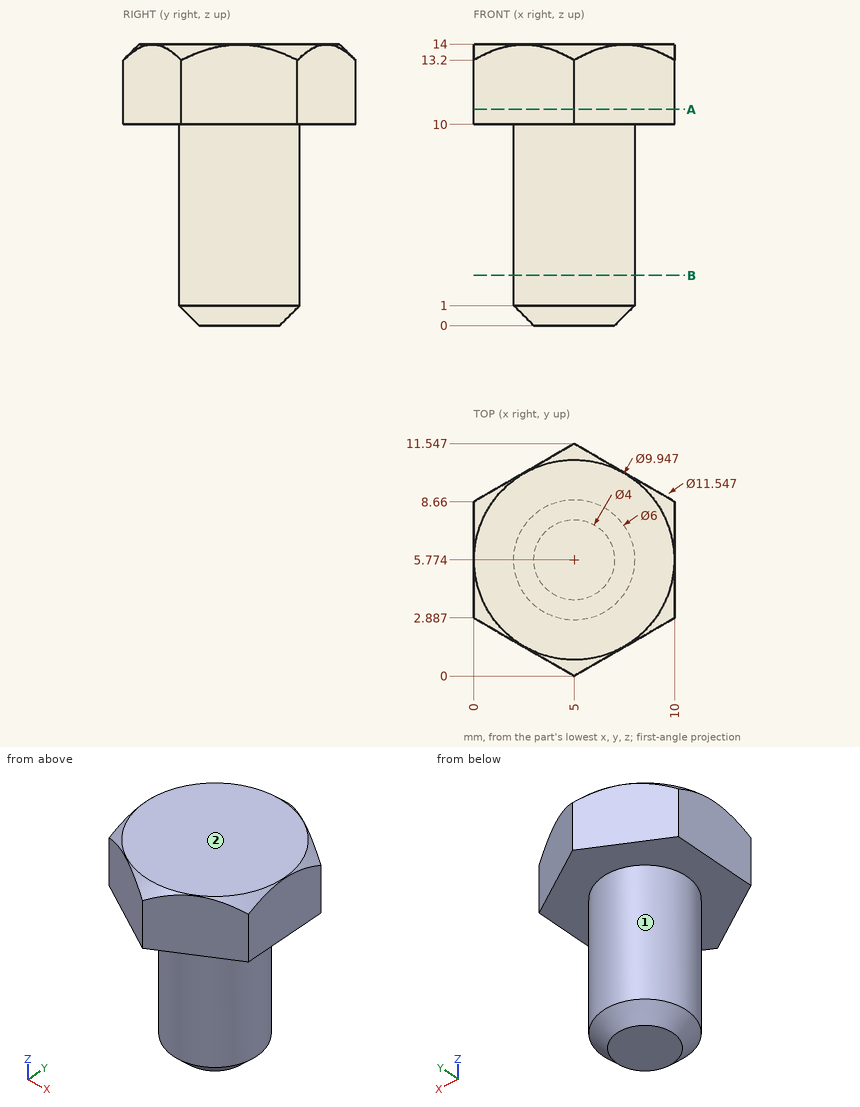
Source: three-view drawing plus pictorial views. Frame: mm from the lowest corner of the part. A direction names the side the tool comes from. Give positions to 0.01 mm unless a question says otherwise; leave off trailing zeros. Order: outer loops, then holes, each group sorted by start corner. A loop starts at its lowest first (then second) coordinate and runs counter-clockwise, first axis right, second up. Notation, with made-up numbers: (-24, 22) - (9, 22) arc R8 cw to (9, 32) - close; hole circle Ø5 at (8.5, 74.25). An arc over 180 degrees is marked (long way). Answer as a JSON object with one key per item and string values. Group by question number.
Q1. First-contact query: pin 1 Ø1 at (y, z) = (5.5, 6.5) entering from -X; pin 2 Ø2 at (x, y) = (2.5, 7.5) entering from -Z. Flat tips, straight axial feed; report the tip coordinate or a pass-through.
Q2. Cut plane A-A, the plane z = 10.75. Output: boundary loops of the cut face in (x, y).
Q3. Cut plane B-B, the plane z = 2.5. Output: boundary loops of the cut face in (x, y).
Q4. Line query: probe 1 along Z at (x, y) = (1, 5.75); probe 2 along Y at (x, z) = (5, 6.5); probe 3 along Y at (x, z) = (1.75, 12.75) (1 decimal). Output: solid intervals per line, ascending.
Q5. Set-up query: the marked faces 1 and 2. Return all of +Z, -Z, +X, -X, +Y, -Y with unobstructed straight access to the full face (end or side cutting, diameter ignored); none if empty.
Results:
{
 "1": {"pin 1": "x = 2", "pin 2": "z = 0.04"},
 "2": {"outline": "(0, 2.89) - (5, 0) - (10, 2.89) - (10, 8.66) - (5, 11.55) - (0, 8.66) - close"},
 "3": {"outline": "circle Ø6 at (5, 5.77)"},
 "4": {"probe 1": "10 to 14", "probe 2": "2.77 to 8.77", "probe 3": "1.9 to 9.7"},
 "5": {"face 1": "-Z", "face 2": "+Z, +X, -X, +Y, -Y"}
}
